Geometry check sheet. Reference: drawing and pictorial views, mm from the part's lowest x, y, z. Give positions to 0.01 mm unless a question says otherwise; leave off trailing zeros. Order: outer loops, then holes, each group sorted by start corner. A loop starts at its lowest first (then second) coordinate and runs counter-clockwise, first axis right, second up. Notation, with made-up numbers: M 88,-10.5 L 131,-10.5 A22 ccw 131,-2.5 Z; hole C 82.25,31.5 d5. An arc over 180 degrees is marked long. Use CSV: the item, a comma, the result in double quotes. Start each with the question number.
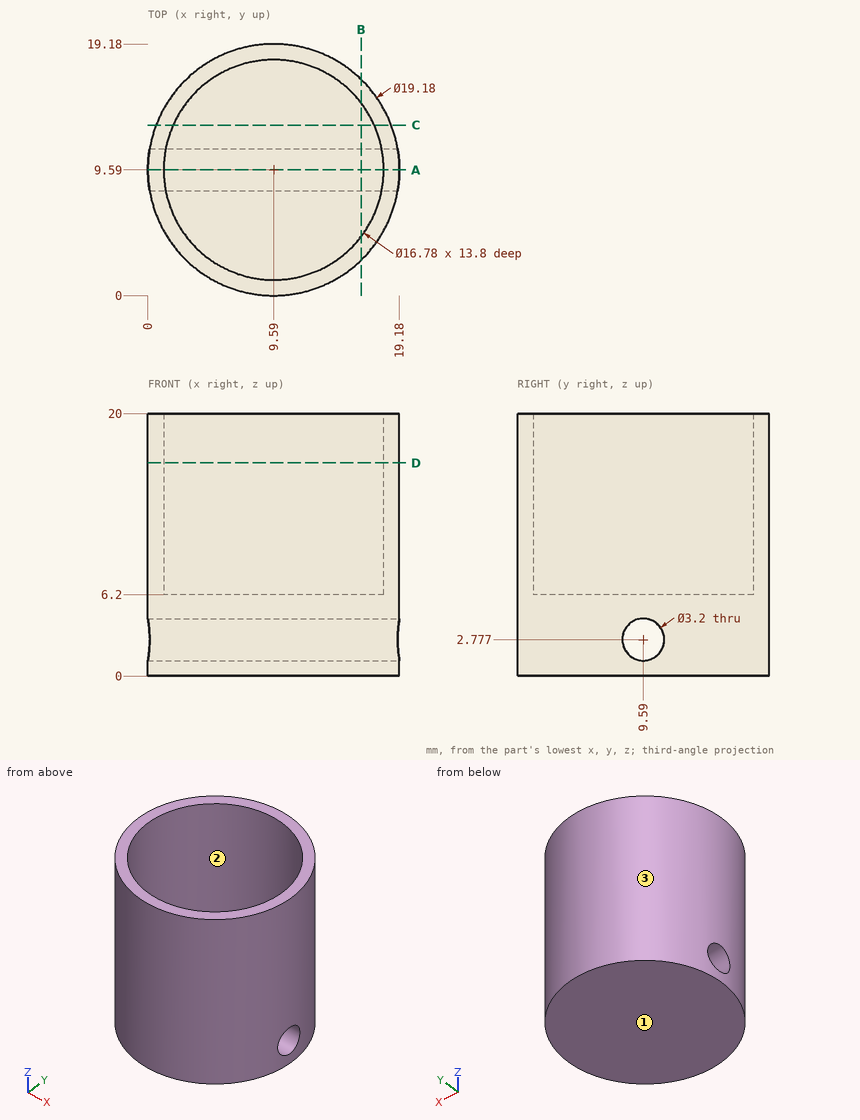
(1) Sectioned sample at B-B on x = 16.25. Record the cut outline in (y, z), then the cut area to 3 significant figures.
(2) Sectioned sample at D-D on z = 16.25. Record the cut outline in (x, y).
(3) Draft check along X on the marked faces 1, 2 and 3. Enter one of: +X half, -X half, draft (parallel to the pull), parting line (faces both ways), or undercut.
(4) Sectioned sample at A-A on y = 9.59. Record the cut outline in (x, z).
(5) Thickness scan on line 1 (Z direction, x = 5.5, y = 9.59); line 2 (Z direction, x = 10.75, y = 4); line 3 (X direction, y = 3.75, z = 6.75) (1 decimal). Record the ranges inside material, lowest first.
(6) Go/stop test with flat-tipped pins: P1, Ø4, axis at y = 6.5, z = 6, coming from the +X side; P2, Ø8, axis at x = 3.5, z = 15, coming from the +Y side; P3, Ø6, axis at x = 7.5, y = 11.5, coming from the +Z side. Record where each tip stops, or that it passes through.
(7) Sectioned sample at C-C on y = 13. Record the cut outline in (x, z), then the cut area to 3 significant figures.
Responses:
1,outline,"M 2.69,0 L 16.49,0 L 16.49,20 L 14.69,20 L 14.69,6.2 L 4.49,6.2 L 4.49,20 L 2.69,20 Z; hole C 9.59,2.78 d3.2"
1,area,"127 mm2"
2,outline,"C 9.59,9.59 d19.18; hole C 9.59,9.59 d16.78"
3,face 1,"draft"
3,face 2,"undercut"
3,face 3,"parting line"
4,outline,"M 0,0 L 19.18,0 L 19.18,1.18 L 0,1.18 Z; M 0,4.38 L 19.18,4.38 L 19.18,20 L 17.98,20 L 17.98,6.2 L 1.2,6.2 L 1.2,20 L 0,20 Z"
5,line 1,"0 to 1.18, 4.38 to 6.2"
5,line 2,"0 to 6.2"
5,line 3,"2 to 3.6, 15.6 to 17.2"
6,P1,"x = 19.12"
6,P2,"y = 18.95"
6,P3,"z = 6.2"
7,outline,"M 0.63,0 L 18.55,0 L 18.55,20 L 17.26,20 L 17.26,6.2 L 1.92,6.2 L 1.92,20 L 0.63,20 Z"
7,area,"147 mm2"
